from build123d import *

# Parameters (mm, degrees)
SUPPORT_PLANE_EXACTLY_20MM_ABOVE_TABLE_DEPTH   = 20
LOW_LOCATING_LIP_0P4MM_CLEARANCE_EACH_SI_START = 20
LOW_LOCATING_LIP_0P4MM_CLEARANCE_EACH_SI_DEPTH = 2


with BuildPart() as part:
    # 草图1 → Support_plane_exactly_20mm_above_table (new body)
    with BuildSketch(Plane.XY):
        Polygon((-61.4, -77.4), (61.4, -77.4), (64.4, -74.4), (64.4, 74.4), (61.4, 77.4), (-61.4, 77.4), (-64.4, 74.4), (-64.4, -74.4), align=None)
        Polygon((-46.8, -60.5), (46.8, -60.5), (47.8, -59.5), (47.8, 59.5), (46.8, 60.5), (-46.8, 60.5), (-47.8, 59.5), (-47.8, -59.5), align=None, mode=Mode.SUBTRACT)
    extrude(amount=SUPPORT_PLANE_EXACTLY_20MM_ABOVE_TABLE_DEPTH)

    # 草图2 → Low_locating_lip_0p4mm_clearance_each_side (add)
    with BuildSketch(Plane.XY.offset(LOW_LOCATING_LIP_0P4MM_CLEARANCE_EACH_SI_START)):
        Polygon((-61.4, -77.4), (61.4, -77.4), (64.4, -74.4), (64.4, 74.4), (61.4, 77.4), (-61.4, 77.4), (-64.4, 74.4), (-64.4, -74.4), align=None)
        Polygon((-59.4, -74.4), (59.4, -74.4), (61.4, -72.4), (61.4, 72.4), (59.4, 74.4), (-59.4, 74.4), (-61.4, 72.4), (-61.4, -72.4), align=None, mode=Mode.SUBTRACT)
    extrude(amount=LOW_LOCATING_LIP_0P4MM_CLEARANCE_EACH_SI_DEPTH)


solid = part.part
For this review, take the finished solid that the model builds, in its own axes (mm). A direction names the side the tool comes from. Give positions to 0.01 mm unless a question says otherwise; leave off trailing zeros. Loops run counter-clockwise (first coordinate to the right, second up) from the corner with the lowest first, then second, coordinate; pieces in that order, holes last. Notation, with made-up numbers: M 49,-36.75 L 59,-36.75 A25 ccw 59,-14.75 Z; hole C 74,62.25 d6. An arc over 180 degrees is marked long. Put each result on its own line as item: value. Start each with the question number.
(1) Wall thickness on L1, parallel to X at y = -13, z = 7.5; L2, parallel to Y at x = -41.5, z = 3.75; L3, parallel to X at y = 21.5, z = 20.5: over which ranges is each line inside the solid? List them lowest first.
(2) For pin 1 (8 mm diameter, centred on x = 51.5, y = -37.5, fed in from -Z), flat-tipped, find the tip position at first contact; note if it passes through.
(3) Add section B-B, the plane x = 23. Write out the cut boundary in (y, z), then the cut area to 3 significant figures.
(4) Machinability: for faces 1 (the flat face through (1, 60.5, 10)), 2 (the flat face through (-1, -77.4, 11)), which of the approach directions +Z, -Z, +X, -X, +Y, -Y give a long, thin tool a straight path to every point of the face, cutting with its end or side? Answer none if there is none.
(5) Add section A-A, the plane z = 3.75. Write out the cut boundary in (x, y).
(6) Add section C-C, the plane y = -65.5. Write out the cut boundary in (x, z).
(7) The part is to be moulded in two halves that separate along Y. For faces 3 (the flat face through (54, 1, 20)), 4 (the flat face through (64.4, -1, 11)), 5 (the flat face through (1, 77.4, 11)), say which applies: +Y half, -Y half, draft (parallel to the pull), parting line (faces both ways), or undercut.
(8) Add section D-D, the plane y = 6.5. Write out the cut boundary in (x, z), then the cut area to 3 significant figures.
Result:
1. L1: x = -64.4 to -47.8, 47.8 to 64.4
1. L2: y = -77.4 to -60.5, 60.5 to 77.4
1. L3: x = -64.4 to -61.4, 61.4 to 64.4
2. pin 1: stops at z = 0
3. outline: M -77.4,0 L -60.5,0 L -60.5,20 L -74.4,20 L -74.4,22 L -77.4,22 Z; M 60.5,0 L 77.4,0 L 77.4,22 L 74.4,22 L 74.4,20 L 60.5,20 Z
3. area: 688 mm^2
4. face 1: +Z, -Z
4. face 2: +Z, -Z, +X, -X, -Y
5. outline: M -64.4,-74.4 L -61.4,-77.4 L 61.4,-77.4 L 64.4,-74.4 L 64.4,74.4 L 61.4,77.4 L -61.4,77.4 L -64.4,74.4 Z; hole M -47.8,-59.5 L -46.8,-60.5 L 46.8,-60.5 L 47.8,-59.5 L 47.8,59.5 L 46.8,60.5 L -46.8,60.5 L -47.8,59.5 Z
6. outline: M -64.4,0 L 64.4,0 L 64.4,22 L 61.4,22 L 61.4,20 L -61.4,20 L -61.4,22 L -64.4,22 Z
7. face 3: undercut
7. face 4: draft
7. face 5: +Y half
8. outline: M -64.4,0 L -47.8,0 L -47.8,20 L -61.4,20 L -61.4,22 L -64.4,22 Z; M 47.8,0 L 64.4,0 L 64.4,22 L 61.4,22 L 61.4,20 L 47.8,20 Z
8. area: 676 mm^2
